Input: part model. Units: mm. Frame: model coordinates. A direction names the side the tool comes from. Give positions to 0.01 mm unless a question says otherwise; leave off trailing zeros. Loops run counter-clockwise (first coordinate to the right, second up) from the corner with the lowest first, then second, coordinate; pieces in that order, holes last. Notation, with made-up numbers: (-18.5, 82) -> (1.5, 82) arc R12 cw to (1.5, 99) -> close; hole circle Ø8 at (-32.75, -8.75). An arc over 180 degrees is marked (long way). Answer in a Markdown table with one row per item. Add a question column.
```python
from build123d import *

# Parameters (mm, degrees)
SKETCH_1_W          = 126
SKETCH_1_H          = 73
SKETCH_1_W_2        = 122
SKETCH_1_H_2        = 70
EXTRUDE_1_DEPTH     = 8
SKETCH_5_W          = 126
SKETCH_5_H          = 73
SKETCH_5_W_2        = 118.02914008
SKETCH_5_H_2        = 66.805819456
EXTRUDE_2_DEPTH     = 2
SKETCH_7_W          = 4
SKETCH_7_H          = 73
EXTRUDE_3_DEPTH     = 2
SKETCH_8_W          = 4
SKETCH_8_H          = 73
EXTRUDE_5_DEPTH     = 2
SKETCH_10_W         = 4
SKETCH_10_H         = 73
EXTRUDE_6_DEPTH     = 5
SKETCH_12_W         = 4
SKETCH_12_H         = 73
EXTRUDE_7_DEPTH     = 3
CUT_EXTRUDE_1_DEPTH = 100.510141559


with BuildPart() as part:
    # 草图1 → 凸台-拉伸1 (new body)
    with BuildSketch(Plane.XY):
        with Locations((22.277543779, 6.299397776)):
            Rectangle(SKETCH_1_W, SKETCH_1_H)
        with Locations((22.29370516, 6.021928133)):
            Rectangle(SKETCH_1_W_2, SKETCH_1_H_2, mode=Mode.SUBTRACT)
    extrude(amount=-EXTRUDE_1_DEPTH)

    # 草图5 → 凸台-拉伸2 (add)
    with BuildSketch(Plane.XY):
        with Locations((22.277543779, 6.299397776)):
            Rectangle(SKETCH_5_W, SKETCH_5_H)
        with Locations((22.456070853, 5.970224549)):
            Rectangle(SKETCH_5_W_2, SKETCH_5_H_2, mode=Mode.SUBTRACT)
    extrude(amount=EXTRUDE_2_DEPTH)

    # 草图7 → 凸台-拉伸3 (add)
    with BuildSketch(Plane(origin=(0, 0, -8), x_dir=(-1, 0, 0), z_dir=(0, 0, -1))):
        with Locations((-87.277543779, 6.299397776)):
            Rectangle(SKETCH_7_W, SKETCH_7_H)
    extrude(amount=-EXTRUDE_3_DEPTH)

    # 草图8 → 凸台-拉伸5 (add)
    with BuildSketch(Plane(origin=(0, 0, -8), x_dir=(-1, 0, 0), z_dir=(0, 0, -1))):
        with Locations((42.722456221, 6.299397776)):
            Rectangle(SKETCH_8_W, SKETCH_8_H)
    extrude(amount=-EXTRUDE_5_DEPTH)

    # 草图10 → 凸台-拉伸6 (add)
    with BuildSketch(Plane.XY.offset(-6)):
        with Locations((87.277543779, 6.299397776)):
            Rectangle(SKETCH_10_W, SKETCH_10_H)
        with Locations((-42.722456221, 6.299397776)):
            Rectangle(SKETCH_10_W, SKETCH_10_H)
    extrude(amount=EXTRUDE_6_DEPTH)

    # 草图12 → 凸台-拉伸7 (add)
    with BuildSketch(Plane.XY.offset(-1)):
        with Locations((-42.722456221, 6.299397776)):
            Rectangle(SKETCH_12_W, SKETCH_12_H)
        with Locations((87.277543779, 6.299397776)):
            Rectangle(SKETCH_12_W, SKETCH_12_H)
    extrude(amount=EXTRUDE_7_DEPTH)

    # 草图13 → 切除-拉伸1 (cut, through all)
    with BuildSketch(Plane.XY.offset(2)):
        with BuildLine():
            ThreePointArc((87.970640893, -27.432685179), (87.531301065, -26.372025007), (86.470640893, -25.932685179))
            Line((86.470640893, -25.932685179), (86.470640893, -27.432685179))
            Line((86.470640893, -27.432685179), (84.970640893, -27.432685179))
            ThreePointArc((84.970640893, -27.432685179), (86.470640893, -28.932685179), (87.970640893, -27.432685179))
        make_face()
        with BuildLine():
            Line((86.470640893, -27.432685179), (86.470640893, -25.932685179))
            ThreePointArc((86.470640893, -25.932685179), (85.409980722, -26.372025007), (84.970640893, -27.432685179))
            Line((84.970640893, -27.432685179), (86.470640893, -27.432685179))
        make_face()
        with BuildLine():
            ThreePointArc((-40.058499187, -27.432685179), (-40.497839015, -26.372025007), (-41.558499187, -25.932685179))
            Line((-41.558499187, -25.932685179), (-41.558499187, -27.432685179))
            Line((-41.558499187, -27.432685179), (-40.058499187, -27.432685179))
        make_face()
        with BuildLine():
            Line((-41.558499187, -27.432685179), (-41.558499187, -25.932685179))
            ThreePointArc((-41.558499187, -25.932685179), (-42.619159359, -28.49334535), (-40.058499187, -27.432685179))
            Line((-40.058499187, -27.432685179), (-41.558499187, -27.432685179))
        make_face()
        with BuildLine():
            Line((-41.558499187, 37.873134277), (-41.558499187, 39.373134277))
            Line((-41.558499187, 39.373134277), (-40.058499187, 39.373134277))
            ThreePointArc((-40.058499187, 39.373134277), (-42.619159359, 40.433794449), (-41.558499187, 37.873134277))
        make_face()
        with BuildLine():
            Line((-40.058499187, 39.373134277), (-41.558499187, 39.373134277))
            Line((-41.558499187, 39.373134277), (-41.558499187, 37.873134277))
            ThreePointArc((-41.558499187, 37.873134277), (-40.497839015, 38.312474105), (-40.058499187, 39.373134277))
        make_face()
        with BuildLine():
            ThreePointArc((87.970640893, 39.373134277), (86.470640893, 40.873134277), (84.970640893, 39.373134277))
            Line((84.970640893, 39.373134277), (86.470640893, 39.373134277))
            Line((86.470640893, 39.373134277), (86.470640893, 37.873134277))
            ThreePointArc((86.470640893, 37.873134277), (87.531301065, 38.312474105), (87.970640893, 39.373134277))
        make_face()
        with BuildLine():
            Line((86.470640893, 39.373134277), (84.970640893, 39.373134277))
            ThreePointArc((84.970640893, 39.373134277), (85.409980722, 38.312474105), (86.470640893, 37.873134277))
            Line((86.470640893, 37.873134277), (86.470640893, 39.373134277))
        make_face()
    extrude(amount=-CUT_EXTRUDE_1_DEPTH, mode=Mode.SUBTRACT)


solid = part.part
```
1) Section C-C on z = -1.75. Output: boundary loops of the cut face in (x, y).
2) Section B-B on y = -18. Output: boundary loops of the cut face in (x, z), and give its area (3 significant figures).
3) Pull-direction query (Y, two-part tool) for faces 1 (the face through (4, -28, 0)), 2 (the face through (22, -29, 2)), 3 (the face through (21, 42.799, -3)), 4 (the face through (83.294, 6, -4)); classes: +Y half, -Y half, draft (parallel to the pull), parting line (faces both ways), or undercut.
4) Material intervals for line 1 along X through (y, z) = (14.5, -1); line 2 along Y through (x, z) = (46, -2.5); line 3 along X through (y, z) = (-26.5, -0.25), sorted ascending.
5) Section A-A on x = 53. Output: boundary loops of the cut face in (y, z).
6) Reachability of faces 5 (the face through (-38.706, 6, -4)), 6 (the face through (21, -30.201, -3)) from +Z, -Z, +X, -X, +Y, -Y: full face, straight path, thin tool, end or side. Return the list, or none.
Working result:
| question | item | result |
|---|---|---|
| 1 | outline | (-44.72, -30.2) -> (89.28, -30.2) -> (89.28, 42.8) -> (-44.72, 42.8) -> close; hole circle Ø3 at (-41.56, -27.43); hole circle Ø3 at (-41.56, 39.37); hole (-38.71, -28.98) -> (83.29, -28.98) -> (83.29, 41.02) -> (-38.71, 41.02) -> close; hole circle Ø3 at (86.47, -27.43); hole circle Ø3 at (86.47, 39.37) |
| 2 | outline | (-44.72, -8) -> (-38.71, -8) -> (-38.71, 0) -> (-36.56, 0) -> (-36.56, 2) -> (-44.72, 2) -> close; (81.47, 0) -> (83.29, 0) -> (83.29, -8) -> (89.28, -8) -> (89.28, 2) -> (81.47, 2) -> close |
| 2 | area | 128 mm2 |
| 3 | face 1 | undercut |
| 3 | face 2 | draft |
| 3 | face 3 | +Y half |
| 3 | face 4 | undercut |
| 4 | line 1 | x = -44.72 to -38.71, 83.29 to 89.28 |
| 4 | line 2 | y = -30.2 to -28.98, 41.02 to 42.8 |
| 4 | line 3 | x = -44.72 to -42.73, -40.38 to -38.71, 83.29 to 85.3, 87.65 to 89.28 |
| 5 | outline | (-30.2, -8) -> (-28.98, -8) -> (-28.98, 0) -> (-27.43, 0) -> (-27.43, 2) -> (-30.2, 2) -> close; (39.37, 0) -> (41.02, 0) -> (41.02, -8) -> (42.8, -8) -> (42.8, 2) -> (39.37, 2) -> close |
| 6 | face 5 | -Z |
| 6 | face 6 | +Z, -Z, +X, -X, -Y |
